Could you check a few things on this model? Use its own coordinates, in mm. Face numbers are marked on the shaded views. A direction names the side the tool comes from. Coordinates: 2 decimals unless noted, no trailing zeros. Write each loop counter-clockwise with the first axis right and the second up, starting at its lowest first coordinate (ties: lowest second). Pieces come first, ordered by that corner, then holes. Notation, with made-up numbers: (23, 9) - (82, 9) arc R25 ccw to (82, 47) - close; hole circle Ø6 at (51.5, 77). An arc over 180 degrees is marked (long way). Write item = value, one per line. Start each with the question number.
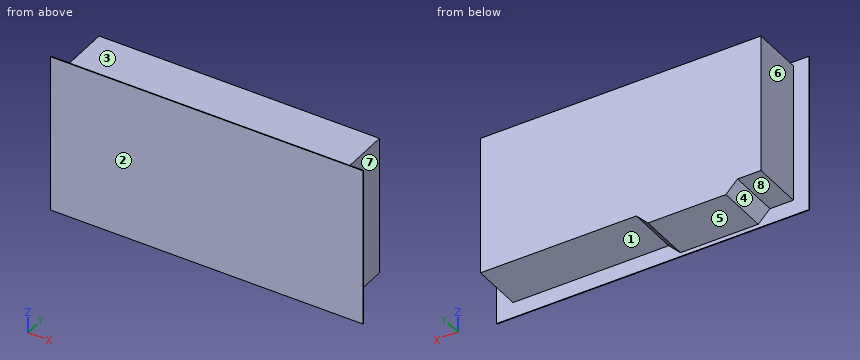
```python
from build123d import *

# Parameters (mm, degrees)
F0_W     = 401
F0_H     = 204
F1_DEPTH = 1
F3_DEPTH = 66


with BuildPart() as f1:
    # F0 (on Front) → F1 (new body)
    with BuildSketch(Plane.XZ):
        with Locations((200.5, 102)):
            Rectangle(F0_W, F0_H)
    extrude(amount=F1_DEPTH)

    # F2 (on face) → F3 (join)
    with BuildSketch(Plane(origin=(0, 0, 0), x_dir=(-1, 0, 0), z_dir=(0, 1, 0))):
        Polygon((-20, 20), (-20, 199), (-380, 199), (-380, 20), (-180, 20), (-165, 5), (-65, 5), (-50, 20), align=None)
    extrude(amount=F3_DEPTH)


solid = f1.part
```
1) If I drill on probe 1 along X at (y, z) = (4.5, 184); probe 2 along Z at (x, y) = (238, 13.5); probe 3 along Z at (x, y) = (64, 27), over which ranges is the centre line in solid material (lowest first)? Write a range as [from, to].
2) Suppose I cut it at A-A on x = 261. Please give me the cut outline in (y, z).
3) Which directions (+Z, -Z, +X, -X, +Y, -Y) give clear straight access to the entire face, cutting with the end or side of a thin tool? Please do the marked faces 1, 2, 3, 4 and 5.
4) Suppose I cut it at B-B on z = 80. Please give me the cut outline in (x, y).
5) For P1, Ø5, axis at y = 57.5, z = 56.5, coming from the -X side; P2, Ø10, axis at x = 333, y = 6, coming from the -Z side; P3, Ø6, axis at y = 6, z = 101, coming from the +X side, each with a flat end and sliding along its axis, tell me the tip position at first contact or that it passes through.
6) Thinking about a two-plate mould opening in X: for the marked faces 6, 7 and 8, which applies, +X half, -X half, draft (parallel to the pull), parting line (faces both ways), or undercut?
Reply:
q1.probe_1 = [20, 380]
q1.probe_2 = [20, 199]
q1.probe_3 = [6, 199]
q2.outline = (-1, 0) - (0, 0) - (0, 20) - (66, 20) - (66, 199) - (0, 199) - (0, 204) - (-1, 204) - close
q3.face_1 = -Z, +X, +Y
q3.face_2 = +Z, -Z, +X, -X, -Y
q3.face_3 = +Z, +X, -X, +Y
q3.face_4 = -Z, -X, +Y
q3.face_5 = -Z, +X, -X, +Y
q4.outline = (0, -1) - (401, -1) - (401, 0) - (380, 0) - (380, 66) - (20, 66) - (20, 0) - (0, 0) - close
q5.P1 = 20
q5.P2 = 20
q5.P3 = 380
q6.face_6 = -X half
q6.face_7 = +X half
q6.face_8 = draft
